For this review, use the dimensioned drawing (mm, ordinates from the lowest corner) and the shaded views. Give positions to 0.01 mm unless a question says otherwise; leave off trailing zeros. Write each loop counter-clockwise with the first axis right and the second up, starting at its lowest first coordinate (ties: lowest second). Pieces come first, ordered by that corner, then holes.
1) For P1, Ø5, axis at y = 120, z = 7.5, coming from the +X side; P2, Ø3, axis at x = 5.5, z = 5.5, coming from the -Y side; P3, Ø2, axis at x = 11, y = 94, coming from the -Z side; P4, Ø4, axis at x = 15.5, z = 6, coming from the +Y side, all flat-tipped, find the tip position at first contact; note any pin that passes through.
2) We need section A-A on x = 5. Give the boundary of the cut face in (y, z), and give its area (3 significant figures).
3) We need section B-B on y = 104. Give the boundary of the cut face in (x, z), and give its area (3 significant figures).
4) Wall thickness on line 1 along Z through (x, y) = (10.5, 92.5); line 2 along Y through (x, z) = (6.75, 8); line 3 along Y through (x, z) = (16, 5.5): over which ranges is each line inside the solid? List them lowest first.
5) We need section C-C on z = 4.25. Give the boundary of the cut face in (x, y), and give its area (3 significant figures).
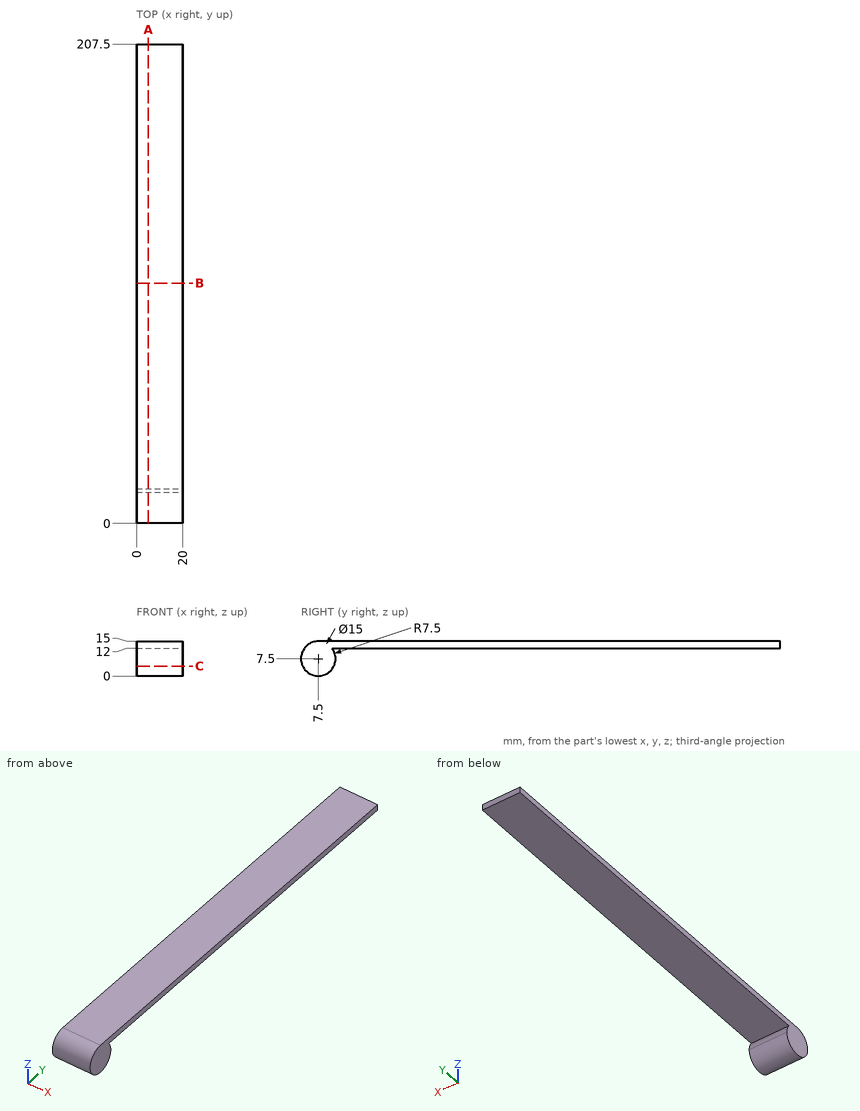
Results list:
1. P1: passes through
1. P2: stops at y = 0.02
1. P3: stops at z = 12
1. P4: stops at y = 15
2. outline: (7.5, 15) arc R7.5 ccw (long way) to (15, 7.5) arc R7.5 ccw to (13.5, 12) - (207.5, 12) - (207.5, 15) - close
2. area: 764 mm2
3. outline: (0, 12) - (20, 12) - (20, 15) - (0, 15) - close
3. area: 60.0 mm2
4. line 1: z = 12 to 15
4. line 2: y = 0.02 to 14.98
4. line 3: y = 0.27 to 14.73
5. outline: (0, 0.74) - (20, 0.74) - (20, 14.26) - (0, 14.26) - close
5. area: 270 mm2
